Source: CAD feature listing. Evaluate the final solid. Frame: model axes, mm. Face numbers are marked on the shaded views. A direction names the side the tool comes from. Give positions to 0.01 mm unless a question says otherwise; leave off trailing zeros. Write each loop counter-clockwise with the first axis right and the second up, starting at its lowest first coordinate (ties: lowest second). Pieces come first, ordered by that corner, then holes. Notation, with made-up numbers: (-8.5, 53) -> (22.5, 53) arc R5 cw to (22.5, 58) -> close; hole circle Ø10 at (71, 54.5). An arc over 180 degrees is marked (long way). Use one line per item in the form item = value. Start each with the question number.
(1) First-contact query: P1, Ø11, axis at x = 211, z = -4.5, coming from the +Y side; P2, Ø1.5, axis at y = 912.5, z = 375, coming from the -X side; P3, Ø16, axis at x = 243, y = 776, coming from the -Z side. Flat tips, straight axial feed; report the tip coordinate or a pass-through.
(2) Cut plane B-B, the plane y = 794. Output: boundary loops of the cut face in (x, z).
(3) Set-up query: the marked faces 1 and 2. Return all of +Z, -Z, +X, -X, +Y, -Y with unobstructed straight access to the full face (end or side cutting, diameter ignored); none if empty.
(4) Material intervals for line 1 along X through (y, z) = (1196, 275.5); line 2 along X through (y, z) = (1630.5, 319); line 3 along Z through (x, y) = (277, 235), sorted ascending. Write a range as from..to.
(5) Cut plane A-A, the plane z = 235. Output: boundary loops of the cut face in (x, y), and give its area (3 significant figures).
from build123d import *

# Parameters (mm, degrees)
SKETCH1_W                = 10.166490401
SKETCH1_H                = 20.32
BOSS_EXTRUDE1_DEPTH      = 450.605251
BOSS_EXTRUDE1_DEPTH_BACK = 10.16
SKETCH2_W                = 40.64
SKETCH2_H                = 88.420284457
CUT_EXTRUDE1_DEPTH       = 1125.982
SKETCH4_W                = 10.16
SKETCH4_H                = 20.292482061
SKETCH4_H_2              = 111.176423169
SKETCH4_H_3              = 88.9
CUT_EXTRUDE2_DEPTH       = 2108.968119463
CUT_EXTRUDE3_REACH       = 2123.564
SKETCH5_W                = 10.16
SKETCH5_H                = 88.9
SKETCH5_H_2              = 55.879999965
SKETCH6_W                = 89.925250809
SKETCH6_H                = 20.32
SKETCH6_W_2              = 90.17
CUT_EXTRUDE4_DEPTH       = 1125.982
SKETCH7_W                = 82.55
SKETCH7_H                = 20.32
SKETCH7_W_2              = 72.39
CUT_EXTRUDE5_DEPTH       = 1125.982
CUT_EXTRUDE6_DEPTH       = 2108.139004111


with BuildPart() as part:
    # Sketch1 → Boss-Extrude1 (new, two sides)
    with BuildSketch(Plane.XY) as boss_extrude1_sk:
        Polygon((291.041413739, 20.32), (280.874923338, 20.32), (205.715298803, 1463.040000035), (205.715298803, 2052.32), (215.881789204, 2052.32), (215.881789204, 1463.040000035), align=None)
        with Locations((285.958168538, 10.16)):
            Rectangle(SKETCH1_W, SKETCH1_H)
        with Locations((210.798544004, 2062.48)):
            Rectangle(SKETCH1_W, SKETCH1_H)
    extrude(amount=BOSS_EXTRUDE1_DEPTH)
    extrude(boss_extrude1_sk.sketch, amount=-BOSS_EXTRUDE1_DEPTH_BACK)

    # Sketch2 → Cut-Extrude1 (cut)
    with BuildSketch(Plane(origin=(605.264675653, -1278.915479685, -1125.851113248), x_dir=(0, -1, 0), z_dir=(-1, 0, 0))):
        Polygon((-3310.915479685, 1576.456364056), (-3310.915479685, 1488.036079599), (-1299.235479685, 1576.456364056), align=None)
        with Locations((-3331.235479685, 1532.246221827)):
            Rectangle(SKETCH2_W, SKETCH2_H)
    extrude(amount=CUT_EXTRUDE1_DEPTH, mode=Mode.SUBTRACT)

    # Sketch4 → Cut-Extrude2 (cut, through all)
    with BuildSketch(Plane(origin=(291.309394939, 15.175990314, 0), x_dir=(0, 0, -1), z_dir=(0.9986457707048434, 0.05202523093009139, 0))):
        with Locations((5.08, -4.99525573)):
            Rectangle(SKETCH4_W, SKETCH4_H)
        with Locations((5.08, 60.739196886)):
            Rectangle(SKETCH4_W, SKETCH4_H_2)
        with Locations((5.08, 249.67740847)):
            Rectangle(SKETCH4_W, SKETCH4_H_3)
        with Locations((5.08, 783.07740847)):
            Rectangle(SKETCH4_W, SKETCH4_H_3)
        with Locations((5.08, 960.87740847)):
            Rectangle(SKETCH4_W, SKETCH4_H_3)
        with Locations((5.08, 1138.67740847)):
            Rectangle(SKETCH4_W, SKETCH4_H_3)
        with Locations((5.08, 1316.47740847)):
            Rectangle(SKETCH4_W, SKETCH4_H_3)
        with Locations((-445.525250809, -4.99525573)):
            Rectangle(SKETCH4_W, SKETCH4_H)
        Polygon((-450.605250809, 5.150985301), (-440.445250809, 5.150985301), (-436.546834031, 93.965468053), (-446.687296633, 94.410572819), align=None)
        Polygon((-411.601545632, 893.740917593), (-401.46108303, 893.295812828), (-397.562666252, 982.11029558), (-407.703128854, 982.555400346), align=None)
        Polygon((-403.804712076, 1071.369883099), (-393.664249474, 1070.924778333), (-389.765832696, 1159.739261086), (-399.906295298, 1160.184365851), align=None)
        Polygon((-396.00787852, 1248.998848604), (-385.867415918, 1248.553743838), (-381.96899914, 1337.368226591), (-392.109461742, 1337.813331357), align=None)
        Polygon((-419.398379188, 716.111952088), (-409.257916585, 715.666847322), (-405.359499808, 804.481330075), (-415.49996241, 804.926434841), align=None)
        Polygon((-455.140613686, 5.150985301), (-450.605250809, 5.150985301), (-446.687296633, 94.410572819), (-450.605250809, 94.410572819), align=None)
        Polygon((-449.818612929, 183.53361819), (-442.788879855, 183.225055572), (-438.890463077, 272.039538325), (-445.920196151, 272.348100943), align=None)
        Polygon((-441.625759495, 361.145200827), (-434.992046299, 360.854021077), (-431.093629521, 449.66850383), (-437.727342717, 449.959683579), align=None)
        Polygon((-434.571427919, 538.806757663), (-427.195212743, 538.482986583), (-423.296795965, 627.297469335), (-430.673011141, 627.621240415), align=None)
        Polygon((-426.54112259, 716.425475174), (-419.398379188, 716.111952088), (-415.49996241, 804.926434841), (-422.642705812, 805.239957927), align=None)
        Polygon((-420.338817864, 894.124430818), (-411.601545632, 893.740917593), (-407.703128854, 982.555400346), (-416.440401086, 982.93891357), align=None)
        Polygon((-415.276210663, 1071.873412266), (-403.804712076, 1071.369883099), (-399.906295298, 1160.184365851), (-411.377793885, 1160.687895019), align=None)
        Polygon((-414.342332906, 1249.80361988), (-396.00787852, 1248.998848604), (-392.109461742, 1337.813331357), (-410.443916128, 1338.618102632), align=None)
        with Locations((5.08, 427.47740847)):
            Rectangle(SKETCH4_W, SKETCH4_H_3)
        with Locations((5.08, 605.27740847)):
            Rectangle(SKETCH4_W, SKETCH4_H_3)
        Polygon((-442.788879855, 183.225055572), (-438.890463077, 272.039538325), (-428.750000475, 271.594433559), (-432.648417253, 182.779950806), align=None)
        Polygon((-434.992046299, 360.854021077), (-431.093629521, 449.66850383), (-420.953166919, 449.223399064), (-424.851583697, 360.408916311), align=None)
        Polygon((-417.054750141, 538.037881817), (-413.156333363, 626.852364569), (-423.296795965, 627.297469335), (-427.195212743, 538.482986583), align=None)
    extrude(amount=-CUT_EXTRUDE2_DEPTH, mode=Mode.SUBTRACT)

    # Cut-Extrude3: up to this face of the body (flat: up to its plane)
    cut_extrude3_end = Plane(part.part.faces().sort_by_distance((205.715298803, 1754.382873748, 182.121056608))[0])
    # Sketch5 → Cut-Extrude3 (cut, up to the picked face)
    with BuildSketch(Plane(origin=(215.881789204, 0, 0), x_dir=(0, 0, -1), z_dir=(1, 0, 0)), mode=Mode.PRIVATE) as cut_extrude3_sk1:
        with Locations((5.08, 2007.87)):
            Rectangle(SKETCH5_W, SKETCH5_H)
    cut_extrude3_tool1 = split(extrude(cut_extrude3_sk1.sketch, amount=-CUT_EXTRUDE3_REACH, mode=Mode.PRIVATE), bisect_by=cut_extrude3_end, keep=Keep.BOTH, mode=Mode.PRIVATE)
    # Sketch5 → Cut-Extrude3 (cut, up to the picked face)
    with BuildSketch(Plane(origin=(215.881789204, 0, 0), x_dir=(0, 0, -1), z_dir=(1, 0, 0)), mode=Mode.PRIVATE) as cut_extrude3_sk2:
        with Locations((5.08, 1830.07)):
            Rectangle(SKETCH5_W, SKETCH5_H)
    cut_extrude3_tool2 = split(extrude(cut_extrude3_sk2.sketch, amount=-CUT_EXTRUDE3_REACH, mode=Mode.PRIVATE), bisect_by=cut_extrude3_end, keep=Keep.BOTH, mode=Mode.PRIVATE)
    # Sketch5 → Cut-Extrude3 (cut, up to the picked face)
    with BuildSketch(Plane(origin=(215.881789204, 0, 0), x_dir=(0, 0, -1), z_dir=(1, 0, 0)), mode=Mode.PRIVATE) as cut_extrude3_sk3:
        with Locations((5.08, 1652.27)):
            Rectangle(SKETCH5_W, SKETCH5_H)
    cut_extrude3_tool3 = split(extrude(cut_extrude3_sk3.sketch, amount=-CUT_EXTRUDE3_REACH, mode=Mode.PRIVATE), bisect_by=cut_extrude3_end, keep=Keep.BOTH, mode=Mode.PRIVATE)
    # Sketch5 → Cut-Extrude3 (cut, up to the picked face)
    with BuildSketch(Plane(origin=(215.881789204, 0, 0), x_dir=(0, 0, -1), z_dir=(1, 0, 0)), mode=Mode.PRIVATE) as cut_extrude3_sk4:
        with Locations((5.08, 1490.980000018)):
            Rectangle(SKETCH5_W, SKETCH5_H_2)
    cut_extrude3_tool4 = split(extrude(cut_extrude3_sk4.sketch, amount=-CUT_EXTRUDE3_REACH, mode=Mode.PRIVATE), bisect_by=cut_extrude3_end, keep=Keep.BOTH, mode=Mode.PRIVATE)
    # Sketch5 → Cut-Extrude3 (cut, up to the picked face)
    with BuildSketch(Plane(origin=(215.881789204, 0, 0), x_dir=(0, 0, -1), z_dir=(1, 0, 0)), mode=Mode.PRIVATE) as cut_extrude3_sk5:
        Polygon((-355.231442512, 1962.99930346), (-351.338294917, 2051.814017969), (-361.488468688, 2052.260153165), (-362.184966352, 2036.370891417), (-362.184966352, 2032), (-365.19852982, 1963.437391374), align=None)
    cut_extrude3_tool5 = split(extrude(cut_extrude3_sk5.sketch, amount=-CUT_EXTRUDE3_REACH, mode=Mode.PRIVATE), bisect_by=cut_extrude3_end, keep=Keep.BOTH, mode=Mode.PRIVATE)
    # Sketch5 → Cut-Extrude3 (cut, up to the picked face)
    with BuildSketch(Plane(origin=(215.881789204, 0, 0), x_dir=(0, 0, -1), z_dir=(1, 0, 0)), mode=Mode.PRIVATE) as cut_extrude3_sk6:
        Polygon((-363.017737701, 1785.369874443), (-359.124590106, 1874.184588952), (-369.102222921, 1874.623140377), (-373.005916021, 1785.80888938), align=None)
    cut_extrude3_tool6 = split(extrude(cut_extrude3_sk6.sketch, amount=-CUT_EXTRUDE3_REACH, mode=Mode.PRIVATE), bisect_by=cut_extrude3_end, keep=Keep.BOTH, mode=Mode.PRIVATE)
    # Sketch5 → Cut-Extrude3 (cut, up to the picked face)
    with BuildSketch(Plane(origin=(215.881789204, 0, 0), x_dir=(0, 0, -1), z_dir=(1, 0, 0)), mode=Mode.PRIVATE) as cut_extrude3_sk7:
        Polygon((-387.19272357, 1463.040000035), (-377.14690292, 1463.040000035), (-374.697180484, 1518.925730918), (-384.716995324, 1519.366136389), align=None)
    cut_extrude3_tool7 = split(extrude(cut_extrude3_sk7.sketch, amount=-CUT_EXTRUDE3_REACH, mode=Mode.PRIVATE), bisect_by=cut_extrude3_end, keep=Keep.BOTH, mode=Mode.PRIVATE)
    # Sketch5 → Cut-Extrude3 (cut, up to the picked face)
    with BuildSketch(Plane(origin=(215.881789204, 0, 0), x_dir=(0, 0, -1), z_dir=(1, 0, 0)), mode=Mode.PRIVATE) as cut_extrude3_sk8:
        Polygon((-370.80403289, 1607.740445426), (-366.910885295, 1696.555159935), (-376.909609122, 1696.994638383), (-380.813302223, 1608.180387386), align=None)
    cut_extrude3_tool8 = split(extrude(cut_extrude3_sk8.sketch, amount=-CUT_EXTRUDE3_REACH, mode=Mode.PRIVATE), bisect_by=cut_extrude3_end, keep=Keep.BOTH, mode=Mode.PRIVATE)
    add(cut_extrude3_tool1.solids().sort_by(Axis((215.881789, 2007.87, -5.08), (-1, 0, 0)))[0], mode=Mode.SUBTRACT)
    add(cut_extrude3_tool2.solids().sort_by(Axis((215.881789, 1830.07, -5.08), (-1, 0, 0)))[0], mode=Mode.SUBTRACT)
    add(cut_extrude3_tool3.solids().sort_by(Axis((215.881789, 1652.27, -5.08), (-1, 0, 0)))[0], mode=Mode.SUBTRACT)
    add(cut_extrude3_tool4.solids().sort_by(Axis((215.881789, 1490.98, -5.08), (-1, 0, 0)))[0], mode=Mode.SUBTRACT)
    add(cut_extrude3_tool5.solids().sort_by(Axis((215.881789, 2007.75713, 358.279909), (-1, 0, 0)))[0], mode=Mode.SUBTRACT)
    add(cut_extrude3_tool6.solids().sort_by(Axis((215.881789, 1829.988805, 366.06296), (-1, 0, 0)))[0], mode=Mode.SUBTRACT)
    add(cut_extrude3_tool7.solids().sort_by(Axis((215.881789, 1491.090003, 380.945152), (-1, 0, 0)))[0], mode=Mode.SUBTRACT)
    add(cut_extrude3_tool8.solids().sort_by(Axis((215.881789, 1652.359856, 373.8598), (-1, 0, 0)))[0], mode=Mode.SUBTRACT)

    # Sketch6 → Cut-Extrude4 (cut)
    with BuildSketch(Plane(origin=(291.041413739, 0, 0), x_dir=(0, 0, -1), z_dir=(1, 0, 0))):
        with Locations((-405.642625404, 10.16)):
            Rectangle(SKETCH6_W, SKETCH6_H)
        with Locations((-225.425, 10.16)):
            Rectangle(SKETCH6_W_2, SKETCH6_H)
        with Locations((-45.085, 10.16)):
            Rectangle(SKETCH6_W_2, SKETCH6_H)
    extrude(amount=-CUT_EXTRUDE4_DEPTH, mode=Mode.SUBTRACT)

    # Sketch7 → Cut-Extrude5 (cut)
    with BuildSketch(Plane(origin=(215.881789204, 0, 0), x_dir=(0, 0, -1), z_dir=(1, 0, 0))):
        with Locations((-31.115, 2062.48)):
            Rectangle(SKETCH7_W, SKETCH7_H)
        with Locations((-180.975, 2062.48)):
            Rectangle(SKETCH7_W_2, SKETCH7_H)
        Polygon((-351.338294917, 2051.814017969), (-351.316115454, 2052.32), (-289.56, 2052.32), (-289.56, 2072.64), (-362.184966352, 2072.64), (-362.184966352, 2036.370891417), (-361.488468688, 2052.260153165), align=None)
    extrude(amount=-CUT_EXTRUDE5_DEPTH, mode=Mode.SUBTRACT)

    # Sketch9 → Cut-Extrude6 (cut, through all)
    with BuildSketch(Plane(origin=(291.309394939, 15.175990314, 0), x_dir=(0, 0, -1), z_dir=(0.9986457707048444, 0.05202523093007474, 0))):
        Polygon((-96.800454295, 369.477574692), (-44.256814481, 443.449817787), (-52.543639813, 449.336079272), (-105.087279627, 375.363836176), align=None)
        Polygon((-201.887733921, 221.533088501), (-149.344094108, 295.505331596), (-157.63091944, 301.39159308), (-210.174559253, 227.419349985), align=None)
        Polygon((-306.975013548, 73.588602309), (-254.431373734, 147.560845405), (-262.718199066, 153.447106889), (-315.26183888, 79.474863794), align=None)
        Polygon((-21.7668071, 588.218839028), (-12.554964696, 592.51040284), (-34.07199968, 638.696721847), (-43.283842083, 634.405158034), align=None)
        Polygon((-55.589034664, 684.883040853), (-77.106069648, 731.069359859), (-86.317912051, 726.777796047), (-64.800877067, 680.591477041), align=None)
    extrude(amount=-CUT_EXTRUDE6_DEPTH, mode=Mode.SUBTRACT)


solid = part.part
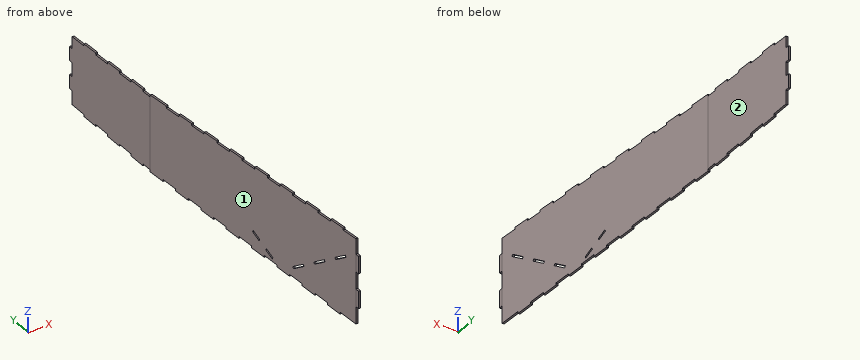
Geometry says:
q1.P1 = 2052.32
q1.P2 = 234.36
q1.P3 = 0
q2.outline = (240.57, 0) -> (250.74, 0) -> (250.74, 406.44) -> (240.57, 406.42) -> close
q3.face_1 = +Z, -Z, -X, -Y
q3.face_2 = +Z, -Z, +X, +Y
q4.line_1 = 219.63..229.79
q4.line_2 = 205.72..215.88
q4.line_3 = 0..431
q5.outline = (205.72, 1463.04) -> (280.87, 20.32) -> (291.04, 20.32) -> (215.88, 1463.04) -> (215.88, 2072.64) -> (205.72, 2072.64) -> close
q5.area = 20,900 mm^2
